from build123d import *

# Parameters (mm, degrees)
EXTRUDE1_DEPTH = 7
FILLET1_R      = 5
SHELL1_T       = -1
EXTRUDE2_DEPTH = 1


with BuildPart() as part:
    # Sketch1 → Extrude1 (new body, symmetric)
    with BuildSketch(Plane.XY):
        Polygon((-10, 0), (10, 0), (10, 2), (0, 6), (-10, 2), align=None)
    extrude(amount=EXTRUDE1_DEPTH, both=True)

    # Fillet1
    fillet1_edges = [part.edges().sort_by_distance(p)[0] for p in [
        (0, 6, 0),
    ]]
    fillet(fillet1_edges, radius=FILLET1_R)

    # Shell1
    shell1_openings = [part.faces().sort_by_distance(p)[0] for p in [
        (0, 0, 0),
    ]]
    offset(amount=SHELL1_T, openings=shell1_openings, kind=Kind.INTERSECTION)

    # Sketch2 → Extrude2 (add, symmetric)
    with BuildSketch(Plane(origin=(0, 0, 0), x_dir=(0, 0, -1), z_dir=(1, 0, 0))):
        Polygon((-6, 0), (-7, 0), (-7, -1.135164807), (-7.75, -1.135164807), (-6, -1.885164807), align=None)
    extrude2 = extrude(amount=EXTRUDE2_DEPTH, both=True)

    # Mirror1: Extrude2 across plane
    add(extrude2.mirror(Plane.XY))


solid = part.part
Verification items for the finished model (mm, model axes). A direction names the side the tool comes from. Coordinates: 2 decimals unless noted, no trailing zeros. Order: outer loops, then holes, each group sorted by start corner. A loop starts at its lowest first (then second) coordinate and runs counter-clockwise, first axis right, second up.
Item 1: Section check D-D, the plane x = -7. Enter the section's corners in (y, z).
Filled in:
outline: (0, -7) - (3.2, -7) - (3.2, 7) - (0, 7) - (0, 6) - (2.12, 6) - (2.12, -6) - (0, -6) - close
Item 2: Depth check by flat-ended pin: pin 1 (1.4 mm diameter, centred on y = -1, z = -7, fed in from -X); pin 2 (1.4 mm diameter, centred on y = -1.5, z = -6.5, fed in from +X); pin 3 (6 mm diameter, centred on x = 8, z = 0.5, fed in from +Y). Enter the tip coordinate at first touch or a pass-through.
Filled in:
pin 1: stops at x = -1
pin 2: stops at x = 1
pin 3: stops at y = 4
Item 3: Material ranges on L1, parallel to Z at x = 1, y = 3; L2, parallel to X at y = 0.25, z = -4.5; L3, parallel to Z at x = -3, y = 4.5, recorded low to high.
Filled in:
L1: z = -7 to -6, 6 to 7
L2: x = -10 to -9, 9 to 10
L3: z = -7 to 7
Item 4: Section check C-C, the plane x = 5.5. Enter the section's corners in (y, z).
Filled in:
outline: (0, -7) - (3.8, -7) - (3.8, 7) - (0, 7) - (0, 6) - (2.72, 6) - (2.72, -6) - (0, -6) - close
Item 5: Access from +Z, -Z, +X, -X, +Y, -Y to the whole of each face (thin tool, end or side, straight path). Record for faces 1 (the face through (1, -0.9, 6.5)), 2 (the face through (0, 2, 7)), 3 (the face through (0, 1, 6)).
Filled in:
face 1: +Z, -Z, +X, -Y
face 2: +Z, +X, -X, +Y
face 3: -Y
Item 6: Section check A-A, the plane y = 1. Enter the section's corners in (x, z), then the cut area to 3 significant figures.
Filled in:
outline: (-10, -7) - (10, -7) - (10, 7) - (-10, 7) - close; hole (-9, -6) - (9, -6) - (9, 6) - (-9, 6) - close
area: 64.0 mm2
Item 7: Section check B-B, the plane z = -4.5. Enter the section's corners in (x, y).
Filled in:
outline: (-10, 0) - (-9, 0) - (-9, 1.32) - (-1.49, 4.33) arc R4 cw to (1.49, 4.33) - (9, 1.32) - (9, 0) - (10, 0) - (10, 2) - (1.86, 5.26) arc R5 ccw to (-1.86, 5.26) - (-10, 2) - close
